from build123d import *

# Parameters (mm, degrees)
F1_DEPTH       = 30
F3_DEPTH       = 50
F7_D           = 5
F7_DEPTH       = 12.7
F7_TIP         = 1.5021515476
F7_ON_F4_D     = 5
F7_ON_F4_DEPTH = 12.7
F7_ON_F4_TIP   = 1.5021515476
F7_ON_F6_D     = 5
F7_ON_F6_DEPTH = 12.7
F7_ON_F6_TIP   = 1.5021515476
F8_R           = 20


with BuildPart() as f1:
    # F0 (on Top) → F1 (new body)
    with BuildSketch(Plane.XY):
        with BuildLine():
            Line((-35, 16.8782217351), (-35, 0))
            Line((-35, 0), (-30, 0))
            Line((-30, 0), (-30, 12.5))
            Line((-30, 12.5), (-20.75, 12.5))
            Line((-20.75, 12.5), (-20.75, 10.37))
            Line((-20.75, 10.37), (-22, 10.37))
            ThreePointArc((-22, 10.37), (-22.5303300859, 10.1503300859), (-22.75, 9.62))
            Line((-22.75, 9.62), (-22.75, 8.12))
            ThreePointArc((-22.75, 8.12), (-22.5303300859, 7.5896699141), (-22, 7.37))
            Line((-22, 7.37), (-13, 7.37))
            ThreePointArc((-13, 7.37), (-12.4696699141, 7.5896699141), (-12.25, 8.12))
            Line((-12.25, 8.12), (-12.25, 9.62))
            ThreePointArc((-12.25, 9.62), (-12.4696699141, 10.1503300859), (-13, 10.37))
            Line((-13, 10.37), (-14.25, 10.37))
            Line((-14.25, 10.37), (-14.25, 12.5))
            Line((-14.25, 12.5), (-5, 12.5))
            Line((-5, 12.5), (-5, 0))
            Line((-5, 0), (0, 0))
            Line((0, 0), (0, 17.5))
            Line((0, 17.5), (2.5, 21.8301270189))
            Line((2.5, 21.8301270189), (-23.4807621135, 36.8301270189))
            Line((-23.4807621135, 36.8301270189), (-35, 16.8782217351))
        make_face()
    extrude(amount=F1_DEPTH)

    # F2 (on face) → F3 (join)
    with BuildSketch(Plane(origin=(10.0777222831, 17.4551270189, 0), x_dir=(-0.8660254038, 0.5, 0), z_dir=(0.5, 0.8660254038, 0))):
        Polygon((13.75, 30), (8.75, 30), (8.75, 0), (38.75, 0), (38.75, 5), (13.75, 5), align=None)
    extrude(amount=F3_DEPTH)

    # F7
    with Locations(Plane.YZ):
        with Locations((0, 15)):
            Hole(F7_D / 2, depth=F7_DEPTH)
            with Locations((0, 0, -(F7_DEPTH + F7_TIP / 2))):  # 118° drill point
                Cone(0, F7_D / 2, F7_TIP, mode=Mode.SUBTRACT)

    # F7 on F4
    with Locations(Plane(origin=(0, 0, 0), x_dir=(1, 0, 0), z_dir=(0, 0, -1))):
        with Locations((-6.4054445662, -41.4054445662), (6.0945554338, -63.0560796608)):
            Hole(F7_ON_F4_D / 2, depth=F7_ON_F4_DEPTH)
            with Locations((0, 0, -(F7_ON_F4_DEPTH + F7_ON_F4_TIP / 2))):  # 118° drill point
                Cone(0, F7_ON_F4_D / 2, F7_ON_F4_TIP, mode=Mode.SUBTRACT)

    # F7 on F6
    with Locations(Plane(origin=(-7.5777222831, 4.375, 0), x_dir=(0.5, 0.8660254038, 0), z_dir=(0.8660254038, -0.5, 0))):
        with Locations((32.6554445662, 17.5), (57.6554445662, 17.5)):
            Hole(F7_ON_F6_D / 2, depth=F7_ON_F6_DEPTH)
            with Locations((0, 0, -(F7_ON_F6_DEPTH + F7_ON_F6_TIP / 2))):  # 118° drill point
                Cone(0, F7_ON_F6_D / 2, F7_ON_F6_TIP, mode=Mode.SUBTRACT)

    # F8
    f8_edges = [f1.edges().sort_by_distance(p)[0] for p in [
        (-35, 16.878222, 15),
        (0, 17.5, 15),
    ]]
    fillet(f8_edges, radius=F8_R)

    # F9: F1 across plane


with BuildPart() as f1_1:
    add(f1.part)
    add(f1.part.mirror(Plane.XZ))


solid = f1_1.part
Check sheet for the modelled part. Datum: model origin and axes. Units: mm. A direction names the side the tool comes from. Round coordinates to 2 decimals unless told otherwise and drop trailing zeros. Loops run counter-clockwise (first coordinate to the right, second up) from the corner with the lowest first, then second, coordinate; pieces in that order, holes last.
1. Sectioned sample at A-A on y = 0. Record the boundary of the cut face in (x, z), and give its area (3 significant figures).
2. Gauge pin test, flat ends, axial feed: pin 1 Ø1.7 at (y, z) = (11, 22) entering from +X; pin 2 Ø6 at (y, z) = (43.5, 9.5) entering from -X; pin 3 Ø0.6 at (y, z) = (-12, 15) entering from -X. Record the tip position at first contact, or that the pin passes through.
3. Set-up check for faces 5 (the cylindrical face through (20.3, -57.74, 17.61)), 6 (the flat face through (-12.5, 30.49, 17.32)), 7 (the flat face through (-10, 12.5, 15)), 8 (the flat face through (-12.5, -30.49, 17.32)), 9 (the flat face through (14.92, 43.34, 15.21)): record each of +Z, -Z, +X, -X, +Y, -Y from which the full face is reachable in a straight line by a thin tool's end or side.
4. Sectioned sample at B-B on x = -17.5. Record the boundary of the cut face in (y, z).
5. Scan lines: probe 1 along Y at (x, z) = (-14, 1); probe 2 along Z at (x, y) = (-1.6, 0); probe 3 along Y at (x, z) = (6, 1.5). Record each from-to range of solid material in increasing order.
6. Mould release check, pull along Y, two halves, no side actions. Record for faces 1 (the flat face through (0, -52, 5)), 2 (the flat face through (24.193, -67.041, 9.514)), 3 (the cylindrical face through (-34.34, 16.62, 15.21)), 4 (the flat face through (14.92, -43.34, 15.21)): released by +Y, released by -Y, zero draft, split by the parting line, or undercut.
7. Sectioned sample at C-C on y = 49. Record the boundary of the cut face in (x, z), and give its area (3 significant figures).
Recorded:
1. outline: (-35, 0) - (-30, 0) - (-30, 30) - (-35, 30) - close; (-5, 0) - (0, 0) - (0, 12.5) - (-5, 12.5) - close; (-5, 17.5) - (0, 17.5) - (0, 30) - (-5, 30) - close
1. area: 275 mm2
2. pin 1: stops at x = 0
2. pin 2: stops at x = 7.51
2. pin 3: stops at x = -35
3. face 5: none
3. face 6: +Z, +Y
3. face 7: +Z, -Z
3. face 8: +Z, -Y
3. face 9: +Z, -Z, +X
4. outline: (-47.19, 0) - (-7.37, 0) - (-7.37, 30) - (-33.38, 30) - (-33.38, 5) - (-47.19, 5) - close; (7.37, 0) - (47.19, 0) - (47.19, 5) - (33.38, 5) - (33.38, 30) - (7.37, 30) - close
5. probe 1: y = -53.25 to -12.5, -10.37 to -7.37, 7.37 to 10.37, 12.5 to 53.25
5. probe 2: z = 0 to 12.5, 17.5 to 30
5. probe 3: y = -77.54 to -65.55, -60.56 to -27.89, 27.89 to 60.56, 65.55 to 77.54
6. face 1: zero draft
6. face 2: released by -Y
6. face 3: released by +Y
6. face 4: undercut
7. outline: (-16.45, 0) - (18.19, 0) - (18.19, 30) - (12.41, 30) - (12.41, 5) - (-16.45, 5) - close
7. area: 318 mm2
